Input: part model. Units: mm. Frame: model coordinates. Give positions to 0.01 mm unless a question says otherwise; leave off trailing zeros. Order: outer loops, then holes, each group sorted by start corner. A loop starts at its lowest first (then second) coordinate and runs counter-clockwise, first axis right, second up. Notation, with made-up numbers: M 88,28 L 140,28 A21 ccw 140,67 Z; hole C -17,17 d9. An arc over 180 degrees is marked long. Use a Markdown table: item, result.
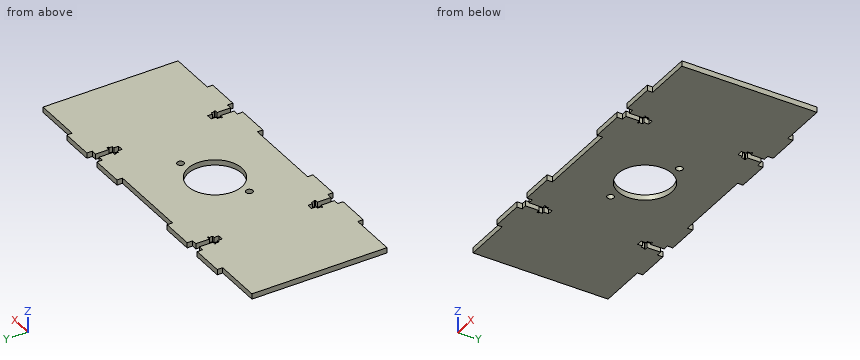
from build123d import *

# Parameters (mm, degrees)
SKETCH1_W           = 250
SKETCH1_H           = 100
BOSS_EXTRUDE1_DEPTH = 4
SKETCH2_W           = 24
SKETCH2_H           = 4
BOSS_EXTRUDE2_DEPTH = 4
CUT_EXTRUDE1_DEPTH  = 10
SKETCH4_R           = 20
SKETCH4_R_2         = 2.5
CUT_EXTRUDE2_DEPTH  = 10


with BuildPart() as part:
    # Sketch1 → Boss-Extrude1 (new body)
    with BuildSketch(Plane.XY):
        Rectangle(SKETCH1_W, SKETCH1_H)
    extrude(amount=BOSS_EXTRUDE1_DEPTH)

    # Sketch2 → Boss-Extrude2 (add)
    with BuildSketch(Plane.XZ.offset(50)):
        with Locations((-78, 2)):
            Rectangle(SKETCH2_W, SKETCH2_H)
        with Locations((-42, 2)):
            Rectangle(SKETCH2_W, SKETCH2_H)
        with Locations((42, 2)):
            Rectangle(SKETCH2_W, SKETCH2_H)
        with Locations((78, 2)):
            Rectangle(SKETCH2_W, SKETCH2_H)
    boss_extrude2 = extrude(amount=BOSS_EXTRUDE2_DEPTH)

    # Mirror1: Boss-Extrude2 across plane
    add(boss_extrude2.mirror(Plane.ZX))

    # Sketch3 → Cut-Extrude1 (cut)
    with BuildSketch(Plane(origin=(0, 0, 0), x_dir=(-1, 0, 0), z_dir=(0, 0, -1))):
        Polygon((-62.1, -50), (-57.9, -50), (-57.9, -40), (-55.5, -40), (-55.5, -39), (-56.25, -39), (-56.25, -36.5), (-57.9, -36.5), (-57.9, -33), (-62.1, -33), (-62.1, -36.5), (-63.75, -36.5), (-63.75, -39), (-64.5, -39), (-64.5, -40), (-62.1, -40), align=None)
        Polygon((57.9, -50), (57.9, -40), (55.5, -40), (55.5, -39), (56.25, -39), (56.25, -36.5), (57.9, -36.5), (57.9, -33), (62.1, -33), (62.1, -36.5), (63.75, -36.5), (63.75, -39), (64.5, -39), (64.5, -40), (62.1, -40), (62.1, -50), align=None)
        Polygon((62.1, 50), (57.9, 50), (57.9, 40), (55.5, 40), (55.5, 39), (56.25, 39), (56.25, 36.5), (57.9, 36.5), (57.9, 33), (62.1, 33), (62.1, 36.5), (63.75, 36.5), (63.75, 39), (64.5, 39), (64.5, 40), (62.1, 40), align=None)
        Polygon((-57.9, 50), (-57.9, 40), (-55.5, 40), (-55.5, 39), (-56.25, 39), (-56.25, 36.5), (-57.9, 36.5), (-57.9, 33), (-62.1, 33), (-62.1, 36.5), (-63.75, 36.5), (-63.75, 39), (-64.5, 39), (-64.5, 40), (-62.1, 40), (-62.1, 50), align=None)
    extrude(amount=-CUT_EXTRUDE1_DEPTH, mode=Mode.SUBTRACT)

    # Sketch4 → Cut-Extrude2 (cut)
    with BuildSketch(Plane(origin=(0, 0, 0), x_dir=(-1, 0, 0), z_dir=(0, 0, -1))):
        Circle(SKETCH4_R)
        with Locations((-25, 10)):
            Circle(SKETCH4_R_2)
        with Locations((25, -10)):
            Circle(SKETCH4_R_2)
    extrude(amount=-CUT_EXTRUDE2_DEPTH, mode=Mode.SUBTRACT)


solid = part.part
1) Cut plane C-C on x = 25. Return loops of the section in (y, z).
Response values:
| item | result |
|---|---|
| outline | M -50,0 L 7.5,0 L 7.5,4 L -50,4 Z; M 12.5,0 L 50,0 L 50,4 L 12.5,4 Z |
2) Cut plane A-A on x = 0. Return loops of the section in (y, z), and give its area (3 significant figures).
Response values:
| item | result |
|---|---|
| outline | M -50,0 L -20,0 L -20,4 L -50,4 Z; M 20,0 L 50,0 L 50,4 L 20,4 Z |
| area | 240 mm² |
3) Cut plane B-B on y = -10. Return loops of the section in (x, z), and give its area (3 significant figures).
Response values:
| item | result |
|---|---|
| outline | M -125,0 L -27.5,0 L -27.5,4 L -125,4 Z; M -22.5,0 L -17.32,0 L -17.32,4 L -22.5,4 Z; M 17.32,0 L 125,0 L 125,4 L 17.32,4 Z |
| area | 841 mm² |
4) Material intervals for line 1 (X direction, y = 38.5, z = 2.3); line 2 (X direction, y = 48.5, z = 3.1); line 3 (Y direction, x = 64, z = 2.5), sorted ascending. Write a range as from..to.
Response values:
| item | result |
|---|---|
| line 1 | x = -125..-63.75, -56.25..56.25, 63.75..125 |
| line 2 | x = -125..-62.1, -57.9..57.9, 62.1..125 |
| line 3 | y = -50..-40, -39..39, 40..50 |
5) Cut plane D-D on z = 2.6. State how many separate pieces and enclosed holes the cut face has, and give its area (3 significant figures).
Response values:
| item | result |
|---|---|
| separate pieces | 1 |
| enclosed holes | 3 |
| area | 24,100 mm² |
6) First-contact query: pin 1 Ø1.2 at (x, z) = (-64.5, 2.5) entering from +Y; pin 2 Ø0.8 at (x, z) = (-62.5, 3) entering from -Y; pin 3 Ø2 at (y, z) = (52, 2) entering from -X. Flat tips, straight axial feed; report the tip coordinate or a pass-through.
Response values:
| item | result |
|---|---|
| pin 1 | stops at y = 50 |
| pin 2 | stops at y = -50 |
| pin 3 | stops at x = -90 |
